Part print with two shaded views. Sizes in mm from the minimum x, y, z corner. Coordinates: 2 decimals unless noted, no trailing zeros. Write each loop counter-clockwise with the first axis right and the second up, starting at its lowest first coordinate (ties: lowest second). Pieces come first, ordered by that corner, then holes. Notation, with made-up numbers: (80, 74) - (119, 74) arc R15 ccw to (119, 90) - close; hole circle Ø6 at (-23, -22.75). An arc over 180 degrees is marked (long way). One line per question, with ' | ' between items. Start each with the question number.
1. Band-saw the part on B-B, the plane y = 8.5. Write the cut outline in (x, z).
2. Band-saw the part on C-C, the plane z = 3.5. Write the cut outline in (x, y).
3. Band-saw the part on D-D, the plane x = 76.5. Write the cut outline in (y, z) (3 decimals).
4. Band-saw the part on A-A, the plane z = 8. Write the cut outline in (x, y).
5. Probe line 1 (Z direction, x = 106.5, y = 7.5); line 2 (Z direction, x = 93, y = 2); line 3 (X direction, y = 3, z = 9.5). List the from-to ranges inside material, lowest first.
6. Flat gauge pins, fed straight in: P1, Ø4, axis at x = 78, z = 5, coming from the -Y side; P2, Ø1.5, axis at x = 59, y = 5, coming from the -Z side; P3, Ø1.1, axis at y = 5, z = 3.5, coming from the -X side. Where does each tip first touch, or does it go through?
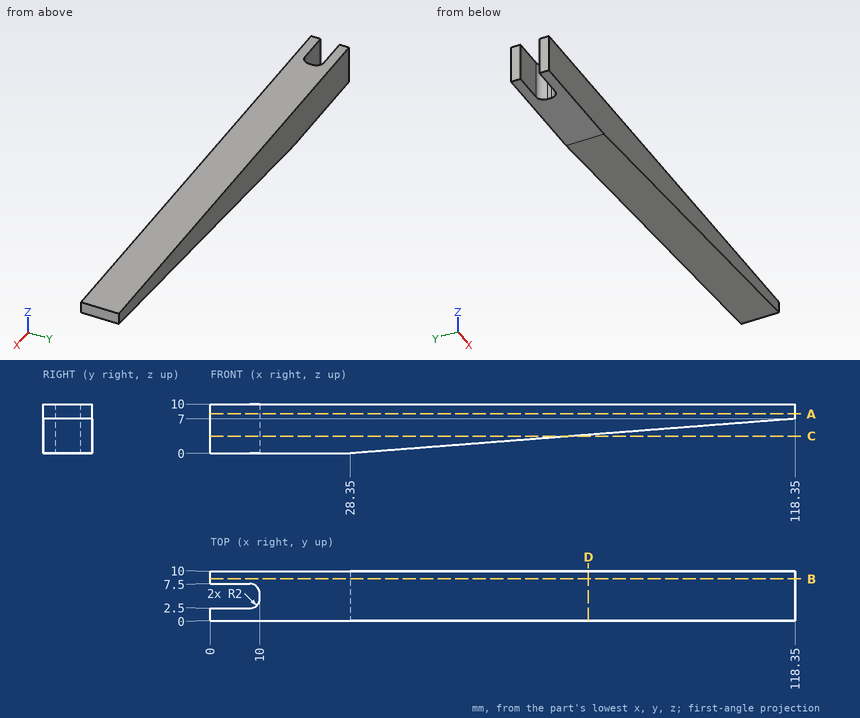
Filled in:
1) outline: (0, 0) - (28.35, 0) - (118.35, 7) - (118.35, 10) - (0, 10) - close
2) outline: (0, 0) - (73.35, 0) - (73.35, 10) - (0, 10) - (0, 7.5) - (8, 7.5) arc R2 cw to (10, 5.5) - (10, 4.5) arc R2 cw to (8, 2.5) - (0, 2.5) - close
3) outline: (0, 3.745) - (10, 3.745) - (10, 10) - (0, 10) - close
4) outline: (0, 0) - (118.35, 0) - (118.35, 10) - (0, 10) - (0, 7.5) - (8, 7.5) arc R2 cw to (10, 5.5) - (10, 4.5) arc R2 cw to (8, 2.5) - (0, 2.5) - close
5) line 1: z = 6.08 to 10 | line 2: z = 5.03 to 10 | line 3: x = 9.32 to 118.35
6) P1: stops at y = 0 | P2: stops at z = 2.33 | P3: stops at x = 10
